Geometry check sheet. Reference: the model listing, model coordinates, mm. Coordinates: 2 decimals unless noted, no trailing zeros. Order: outer loops, then holes, each group sorted by start corner. A loop starts at its lowest first (then second) coordinate and runs counter-clockwise, first axis right, second up. Notation, with made-up numbers: (27, 45) - (75, 45) arc R30 cw to (75, 72) - close; hole circle Ø2 at (5.5, -33). An arc over 180 degrees is marked (long way). Put each result on its own line as item: value.
Autodesk Inventor part; units mm, degrees
ref_plane "YZ Plane" through (0, 0, 0) normal (1, 0, 0) x (0, 1, 0)
ref_plane "XZ Plane" through (0, 0, 0) normal (0, 1, 0) x (-1, 0, 0)
ref_plane "XY Plane" through (0, 0, 0) normal (0, 0, 1) x (1, 0, 0)
sketch "Esboço1" plane through (0, 0, 0) normal (1, 0, 0) x (0, 1, 0)
  line L0 (19.0364, -63.7913) -> (-150.9636, -63.7913)
  line L1 (-150.9636, -63.7913) -> (-150.9636, -51.7913)
  line L2 (19.0364, -51.7913) -> (19.0364, -63.7913)
  circle A0 centre (-146.5949, -57.7913) radius 2.5
  line L3 (19.0364, -51.7913) -> (-150.9636, -51.7913)
  circle A1 centre (-136.5949, -57.7913) radius 2.5
  circle A2 centre (-126.5949, -57.7913) radius 2.5
  circle A3 centre (-116.5949, -57.7913) radius 2.5
  circle A4 centre (-106.5949, -57.7913) radius 2.5
  circle A5 centre (-96.5949, -57.7913) radius 2.5
  circle A6 centre (-86.5949, -57.7913) radius 2.5
  circle A7 centre (-76.5949, -57.7913) radius 2.5
  circle A8 centre (-66.5949, -57.7913) radius 2.5
  circle A9 centre (-56.5949, -57.7913) radius 2.5
  circle A10 centre (-46.5949, -57.7913) radius 2.5
  circle A11 centre (-36.5949, -57.7913) radius 2.5
  circle A12 centre (-26.5949, -57.7913) radius 2.5
  circle A13 centre (-16.5949, -57.7913) radius 2.5
  circle A14 centre (-6.5949, -57.7913) radius 2.5
  circle A15 centre (3.4051, -57.7913) radius 2.5
  circle A16 centre (13.4051, -57.7913) radius 2.5
  point P0 (0, 0)
  dimension "d2" = 12
  dimension "d3" = 170
  dimension "d4" = 5
  dimension "d10" = 10
extrude "Extrusão1" add sketch "Esboço1" along normal blind 1
properties part number "aste2"
Q1. Section check B-B on x = 0.4. State how many separate pieces and enclosed holes the cut face has, then the cut area to 3 significant figures.
Answer block:
separate pieces: 1
enclosed holes: 17
area: 1,710 mm^2
Q2. Thickness scan on L1, parallel to Z at x = 0.7, y = -107; L2, parallel to Z at x = 0.4, y = -15.5. Record the ranges inside material, lowest first. Write a range as [from, to].
Answer block:
L1: z = [-63.79, -60.26], [-55.32, -51.79]
L2: z = [-63.79, -60.04], [-55.54, -51.79]
Q3. Section check C-C on y = -117.5. Record the boundary of the cut face in (x, z), then the cut area to 3 significant figures.
Answer block:
outline: (0, -63.79) - (1, -63.79) - (1, -60.12) - (0, -60.12) - close; (0, -55.46) - (1, -55.46) - (1, -51.79) - (0, -51.79) - close
area: 7.34 mm^2
Q4. Section check A-A on y = -77. Record the boundary of the cut face in (x, z).
Answer block:
outline: (0, -63.79) - (1, -63.79) - (1, -60.26) - (0, -60.26) - close; (0, -55.32) - (1, -55.32) - (1, -51.79) - (0, -51.79) - close
Q5. Depth check by flat-ended pin: pin 1 Ø6.5 at (y, z) = (-96.59, -57.79) entering from +X; pin 2 Ø3 at (y, z) = (-126.59, -57.79) entering from -X. Enter the tip coordinate at first touch or a pass-through.
Answer block:
pin 1: stops at x = 1
pin 2: passes through
Q6. Draft check along Z on faces 1 (the cylindrical face through (0.5, -144.3, -56.8)), 2 (the cylindrical face through (0.5, -98.6, -56.3)), 3 (the flat face through (1, -67.2, -60.4)). Enter one of: pulls with the +Z half, pulls with the -Z half, needs draft (parallel to the pull), parting line crosses it, or undercut.
Answer block:
face 1: undercut
face 2: undercut
face 3: needs draft
